Geometry check sheet. Reference: the model listing, model coordinates, mm. A direction names the side the tool comes from. Give positions to 0.01 mm unless a question says otherwise; leave off trailing zeros. Order: outer loops, then holes, each group sorted by start corner. A loop starts at its lowest first (then second) coordinate and runs counter-clockwise, first axis right, second up.
from build123d import *

# Parameters (mm, degrees)
SKETCH1_W           = 171.45
SKETCH1_H           = 36.83
BOSS_EXTRUDE1_DEPTH = 3.175
SKETCH2_W           = 12.7
SKETCH2_H           = 3.175
SKETCH2_W_2         = 50.8
BOSS_EXTRUDE2_DEPTH = 3.175
SKETCH3_W           = 42.418
SKETCH3_H           = 12.7
CUT_EXTRUDE1_DEPTH  = 3.175
SKETCH5_W           = 17.018
SKETCH5_H           = 12.7
BOSS_EXTRUDE3_DEPTH = 3.175
SKETCH6_W           = 3.175
SKETCH6_H           = 17.78
BOSS_EXTRUDE4_DEPTH = 3.175
SKETCH7_W           = 59.348335251
SKETCH7_H           = 25.17302984
BOSS_EXTRUDE5_DEPTH = 3.175


with BuildPart() as part:
    # Sketch1 → Boss-Extrude1 (new body)
    with BuildSketch(Plane(origin=(0, 0, 0), x_dir=(1, 0, 0), z_dir=(0, 1, 0))):
        with Locations((85.725, 18.415)):
            Rectangle(SKETCH1_W, SKETCH1_H)
    extrude(amount=BOSS_EXTRUDE1_DEPTH)

    # Sketch2 → Boss-Extrude2 (add)
    with BuildSketch(Plane(origin=(0, 3.175, 0), x_dir=(1, 0, 0), z_dir=(0, 1, 0))):
        with Locations((15.875, -1.5875)):
            Rectangle(SKETCH2_W, SKETCH2_H)
        with Locations((41.275, -1.5875)):
            Rectangle(SKETCH2_W, SKETCH2_H)
        with Locations((85.725, -1.5875)):
            Rectangle(SKETCH2_W_2, SKETCH2_H)
        with Locations((130.175, -1.5875)):
            Rectangle(SKETCH2_W, SKETCH2_H)
        with Locations((155.575, -1.5875)):
            Rectangle(SKETCH2_W, SKETCH2_H)
    boss_extrude2 = extrude(amount=-BOSS_EXTRUDE2_DEPTH)

    # Sketch3 → Cut-Extrude1 (cut)
    with BuildSketch(Plane(origin=(0, 3.175, 0), x_dir=(1, 0, 0), z_dir=(0, 1, 0))):
        with Locations((88.646, 9.525)):
            Rectangle(SKETCH3_W, SKETCH3_H)
    extrude(amount=-CUT_EXTRUDE1_DEPTH, mode=Mode.SUBTRACT)

    # Sketch5 → Boss-Extrude3 (add)
    with BuildSketch(Plane(origin=(0, 3.175, 0), x_dir=(1, 0, 0), z_dir=(0, 1, 0))):
        with Locations((89.916, 9.525)):
            Rectangle(SKETCH5_W, SKETCH5_H)
    extrude(amount=-BOSS_EXTRUDE3_DEPTH)

    # Sketch6 → Boss-Extrude4 (add)
    with BuildSketch(Plane(origin=(0, 3.175, 0), x_dir=(1, 0, 0), z_dir=(0, 1, 0))):
        with Locations((-1.5875, 18.415)):
            Rectangle(SKETCH6_W, SKETCH6_H)
        with Locations((173.0375, 18.415)):
            Rectangle(SKETCH6_W, SKETCH6_H)
    extrude(amount=-BOSS_EXTRUDE4_DEPTH)

    # Mirror1: Boss-Extrude2 across plane
    add(boss_extrude2.mirror(Plane(origin=(0, 0, -18.415), x_dir=(1, 0, 0), z_dir=(0, 0, -1))))

    # Sketch7 → Boss-Extrude5 (add)
    with BuildSketch(Plane(origin=(0, 3.175, 0), x_dir=(1, 0, 0), z_dir=(0, 1, 0))):
        with Locations((85.808354404, 13.913862214)):
            Rectangle(SKETCH7_W, SKETCH7_H)
    extrude(amount=-BOSS_EXTRUDE5_DEPTH)


solid = part.part
Item 1: Sectioned sample at A-A (z = -30). Enter the section's corners in (x, y) (3 decimals), and give its area (3 significant figures).
Reported:
outline: (0, 0) - (171.45, 0) - (171.45, 3.175) - (0, 3.175) - close
area: 544 mm2
Item 2: Gauge pin test, flat ends, axial feed: pin 1 (1 mm diameter, centred on y = 1, z = 2, fed in from +X) (3 decimals); pin 2 (1.6 mm diameter, centred on x = 119.5, y = 2, fed in from +Z); pin 3 (1.6 mm diameter, centred on y = 2, z = 1.5, fed in from -X) (3 decimals); pin 4 (12 mm diameter, centred on x = 48.5, z = -10, fed in from -Y). Record the tip position at first contact, or that the pin passes through.
Reported:
pin 1: stops at x = 161.925
pin 2: stops at z = 0
pin 3: stops at x = 9.525
pin 4: stops at y = 0
Item 3: Draft check along X on faces 5 (the flat face through (47.625, 2, 2)), 6 (the flat face through (9.525, 2, -38)), 7 (the flat face through (123.825, 2, -38)), 8 (the flat face through (161.925, 2, -38)). Enter one of: released by +X, released by -X, zero draft, split by the parting line, or undercut.
Reported:
face 5: undercut
face 6: released by -X
face 7: undercut
face 8: released by +X
Item 4: Scan lines: L1, parallel to X at y = 0.95, z = 1 (3 decimals); L2, parallel to Z at x = 143, y = 2.05; L3, parallel to X at y = 0.5, z = -0.5. Record each from-to range of solid material in increasing order.
Reported:
L1: x = 9.525 to 22.225, 34.925 to 47.625, 60.325 to 111.125, 123.825 to 136.525, 149.225 to 161.925
L2: z = -36.83 to 0
L3: x = 0 to 171.45
Item 5: Sectioned sample at B-B (x = 147). Enter the section's corners in (y, z) (3 decimals).
Reported:
outline: (0, -36.83) - (3.175, -36.83) - (3.175, 0) - (0, 0) - close
Item 6: Set-up check for faces 1 (the flat face through (-2, 2, -9.525)), 2 (the flat face through (54, 2, 0)), 3 (the flat face through (143, 2, -36.83)), 4 (the flat face through (85, 2, 3.175)): record each of +Z, -Z, +X, -X, +Y, -Y from which the full face is reachable in a straight line by a thin tool's end or side.
Reported:
face 1: +Z, -X, +Y, -Y
face 2: +Z, +Y, -Y
face 3: -Z, +Y, -Y
face 4: +Z, +X, -X, +Y, -Y
